Source: CAD feature listing. Evaluate the final solid. Frame: model axes, mm. A direction names the side the tool comes from. Round coordinates to 2 decimals unless told otherwise and drop trailing zeros. Loops run counter-clockwise (first coordinate to the right, second up) from the corner with the lowest first, then second, coordinate; pieces in that order, holes last. Notation, with made-up numbers: (76.5, 20.25) -> (92.5, 20.25) arc R27 ccw to (92.5, 47.25) -> close; hole circle Ø6 at (86.25, 86.25). An arc over 180 degrees is marked (long way). Return JSON: item names as keys, results as strings. Group by question number.
```python
from build123d import *

# Parameters (mm, degrees)
SKETCH2_W           = 75
SKETCH2_H           = 50
BOSS_EXTRUDE1_DEPTH = 101.6
CUT_EXTRUDE1_DEPTH  = 101.6
CUT_EXTRUDE2_DEPTH  = 101.6
SKETCH5_W           = 20
SKETCH5_H           = 40
CUT_EXTRUDE3_DEPTH  = 10
SKETCH6_W           = 20
SKETCH6_H           = 40
CUT_EXTRUDE4_DEPTH  = 10


with BuildPart() as part:
    # Sketch2 → Boss-Extrude1 (new body)
    with BuildSketch(Plane.XY):
        with Locations((-3.307692308, -6.81353022)):
            Rectangle(SKETCH2_W, SKETCH2_H)
    extrude(amount=BOSS_EXTRUDE1_DEPTH)

    # Sketch3 → Cut-Extrude1 (cut)
    with BuildSketch(Plane(origin=(0, 18.18646978, 0), x_dir=(1, 0, 0), z_dir=(0, 1, 0))):
        Polygon((-40.807692308, -7.5), (-20.807692308, -7.5), (-7.507692308, -20.8), (-7.507692308, -80.8), (-20.807692308, -94.1), (-40.807692308, -94.1), align=None)
    extrude(amount=-CUT_EXTRUDE1_DEPTH, mode=Mode.SUBTRACT)

    # Sketch4 → Cut-Extrude2 (cut)
    with BuildSketch(Plane(origin=(0, 18.18646978, 0), x_dir=(1, 0, 0), z_dir=(0, 1, 0))):
        Polygon((34.192307692, -94.1), (14.192307692, -94.1), (0.892307692, -80.8), (0.892307692, -20.8), (14.192307692, -7.5), (34.192307692, -7.5), align=None)
    extrude(amount=-CUT_EXTRUDE2_DEPTH, mode=Mode.SUBTRACT)

    # Sketch5 → Cut-Extrude3 (cut)
    with BuildSketch(Plane.XY.offset(101.6)):
        with Locations((24.192307692, -6.81353022)):
            Rectangle(SKETCH5_W, SKETCH5_H)
    extrude(amount=-CUT_EXTRUDE3_DEPTH, mode=Mode.SUBTRACT)

    # Sketch6 → Cut-Extrude4 (cut)
    with BuildSketch(Plane.XY.offset(101.6)):
        with Locations((-30.807692308, -6.81353022)):
            Rectangle(SKETCH6_W, SKETCH6_H)
    extrude(amount=-CUT_EXTRUDE4_DEPTH, mode=Mode.SUBTRACT)


solid = part.part
```
(1) Pin query (flat end, axial travel): pin 1 (5.5 mm diameter, centred on x = -30, y = 15.5, fed in from -Z); pin 2 (6 mm diameter, centred on x = -30.5, y = -4.5, fed in from +Z); pin 3 (5 mm diameter, centred on y = 1, z = 81, fed in from +X); pin 4 (2 mm diameter, centred on y = -3, z = 97, fed in from +X). Return the tip coordinate at first contact, or that it passes through.
(2) Set-up query: faces 5 (the face through (-31, 13.186, 98)), 6 (the face through (14.192, -7, 98)), 7 (the face through (-31, 16, 94.1)), 8 (the face through (24, -29, 94.1)). Return all of +Z, -Z, +X, -X, +Y, -Y with unobstructed straight access to the full face (end or side cutting, diameter ignored); none if empty.
(3) Cut plane D-D (z = 44.5). Return loops of the section in (x, y), and give its area (3 significant figures).
(4) Cut plane C-C (x = -22). Return loops of the section in (y, z).
(5) Cut plane B-B (y = -1). Return loops of the section in (x, z).
(6) Ray query, line 1 (X direction, y = -9.5, z = 33.5); line 2 (Z direction, x = 28, y = -25.5); line 3 (Z direction, x = 4, y = -27). Return the intervals inside material, ascending.
(7) Cut plane A-A (x = 5). Return loops of the section in (y, z), and give its area (3 significant figures).
(8) Mould query, pull axis Y, two halves, no side actions, for faces 1 (the face through (24, -6, 7.5)), 2 (the face through (-31, -26.814, 98)), 3 (the face through (-6, -31.814, 51)), 4 (the face through (-6, 18.186, 51)). Classes: released by +Y, released by -Y, zero draft, split by the parting line, or undercut.
Answers follow:
{
 "1": {"pin 1": "z = 0", "pin 2": "z = 7.5", "pin 3": "x = 3.59", "pin 4": "x = 14.19"},
 "2": {"face 5": "+Z, -X", "face 6": "+Z, +X", "face 7": "-X, +Y, -Y", "face 8": "+X, +Y, -Y"},
 "3": {"outline": "(-7.51, -31.81) -> (0.89, -31.81) -> (0.89, 18.19) -> (-7.51, 18.19) -> close", "area": "420 mm^2"},
 "4": {"outline": "(-31.81, 0) -> (18.19, 0) -> (18.19, 7.5) -> (-31.81, 7.5) -> close; (-31.81, 94.1) -> (-26.81, 94.1) -> (-26.81, 101.6) -> (-31.81, 101.6) -> close; (13.19, 94.1) -> (18.19, 94.1) -> (18.19, 101.6) -> (13.19, 101.6) -> close"},
 "5": {"outline": "(-40.81, 0) -> (34.19, 0) -> (34.19, 7.5) -> (14.19, 7.5) -> (0.89, 20.8) -> (0.89, 80.8) -> (14.19, 94.1) -> (14.19, 101.6) -> (-20.81, 101.6) -> (-20.81, 94.1) -> (-7.51, 80.8) -> (-7.51, 20.8) -> (-20.81, 7.5) -> (-40.81, 7.5) -> close"},
 "6": {"line 1": "-7.51 to 0.89", "line 2": "0 to 7.5", "line 3": "0 to 17.69, 83.91 to 101.6"},
 "7": {"outline": "(-31.81, 0) -> (18.19, 0) -> (18.19, 16.69) -> (-31.81, 16.69) -> close; (-31.81, 84.91) -> (18.19, 84.91) -> (18.19, 101.6) -> (-31.81, 101.6) -> close", "area": "1,670 mm^2"},
 "8": {"face 1": "zero draft", "face 2": "undercut", "face 3": "released by -Y", "face 4": "released by +Y"}
}
